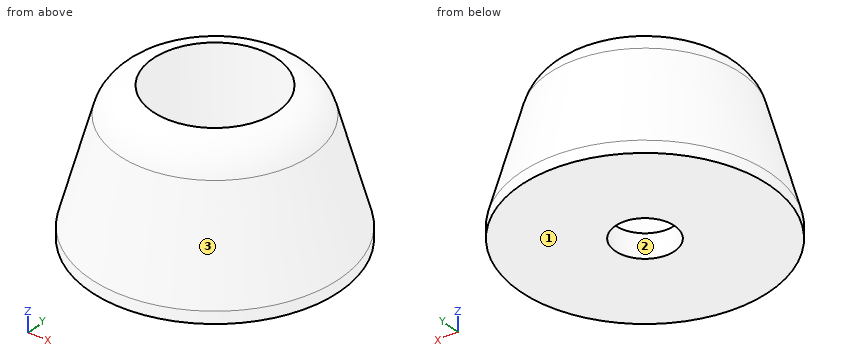
```python
from build123d import *

# Parameters (mm, degrees)
F0_R      = 10.5
F1_DEPTH  = 1
F1_FACE_R = 10.5
F3_R      = 7.5
F5_R      = 2.5
F6_DEPTH  = 12
F7_R      = 5.25
F8_DEPTH  = 10


# Not quite as in the source:
# - a fillet or chamfer that OpenCascade refuses, or shapes differently, is made with other operations: its cross-section is extruded or revolved along the edge and cut away or added


with BuildPart() as f1:
    # F0 (on Top) → F1 (new body)
    with BuildSketch(Plane.XY):
        Circle(F0_R)
    extrude(amount=F1_DEPTH)

    # F1_face (on face) → F4 section 0
    with BuildSketch(Plane.XY.offset(1)):
        Circle(F1_FACE_R)
    # F3 (on offset) → F4 section 1
    with BuildSketch(Plane.XY.offset(12)):
        Circle(F3_R)
    loft()

    # F5 (on Top) → F6 (cut, through all)
    with BuildSketch(Plane.XY):
        Circle(F5_R)
    extrude(amount=F6_DEPTH, mode=Mode.SUBTRACT)

    # F7 (on offset) → F8 (cut)
    with BuildSketch(Plane.XY.offset(12)):
        Circle(F7_R)
    extrude(amount=-F8_DEPTH, mode=Mode.SUBTRACT)

    # F9: fillet of radius 3.0968632265 on 1 edges, made by hand

    # F9_s1 → F9_t2 (revolve, cut)
    with BuildSketch(Plane.XZ):
        with BuildLine():
            ThreePointArc((8.1217780062, 9.7201473108), (7.0595697228, 11.3307742745), (5.25, 12))
            Line((5.25, 12), (7.5, 12))
            Line((7.5, 12), (8.1217780062, 9.7201473108))
        make_face()
    revolve(axis=Axis((0, 0, 12), (0, 0, 1)), mode=Mode.SUBTRACT)


solid = f1.part
```
Model file for the job. Use its own axes, mm. Face numbers are marked on the shaded views. Round coordinates to 2 decimals unless told otherwise and drop trailing zeros. Order: outer loops, then holes, each group sorted by start corner. A loop starts at its lowest first (then second) coordinate and runs counter-clockwise, first axis right, second up. Notation, with made-up numbers: (-15, 52) -> (14, 52) arc R25 ccw to (14, 88) -> close; hole circle Ø6 at (-29.75, -30.75). An arc over 180 degrees is marked (long way). Use one line per item in the form item = value.
Item 1: Drill centre lines: line 1 (Y direction, x = 0, z = 6.5); line 2 (Y direction, x = 1.25, z = 3.75); line 3 (X direction, y = 2, z = 11). Where is each one in solid material? Low to high.
Returned:
line_1 = -9 to -5.25, 5.25 to 9
line_2 = -9.67 to -5.1, 5.1 to 9.67
line_3 = -7.14 to -4.85, 4.85 to 7.14
Item 2: Pull direction X, two halves, no side cores. Call the marked faces 1, 2 and 3: released by +X, released by -X, zero draft, split by the parting line, or undercut.
Returned:
face_1 = zero draft
face_2 = undercut
face_3 = split by the parting line
Item 3: Flat gauge pins, fed straight in: pin 1 Ø1 at (x, z) = (-3, 4.5) entering from -Y; pin 2 Ø1 at (x, z) = (-4, 7.5) entering from -Y; pin 3 Ø5 at (y, z) = (-4.5, 8) entering from -X. Where does each tip first touch, or does it go through?
Returned:
pin_1 = -9.27
pin_2 = -8.04
pin_3 = -8.65
Item 4: Cut at A-A, the plane x = 0. Write the cut outline in (y, z), and give its area (3 significant figures).
Returned:
outline = (-10.5, 0) -> (-2.5, 0) -> (-2.5, 2) -> (-5.25, 2) -> (-5.25, 12) arc R3.1 ccw to (-8.12, 9.72) -> (-10.5, 1) -> close; (2.5, 0) -> (10.5, 0) -> (10.5, 1) -> (8.12, 9.72) arc R3.1 ccw to (5.25, 12) -> (5.25, 2) -> (2.5, 2) -> close
area = 102 mm^2
Item 5: Cut at C-C, the plane z = 6.75. Write the cut outline in (x, y).
Returned:
outline = circle Ø17.86 at (0, 0); hole circle Ø10.5 at (0, 0)
Item 6: Cut at B-B, the plane z = 2.5. Write the cut outline in (x, y).
Returned:
outline = circle Ø20.18 at (0, 0); hole circle Ø10.5 at (0, 0)
